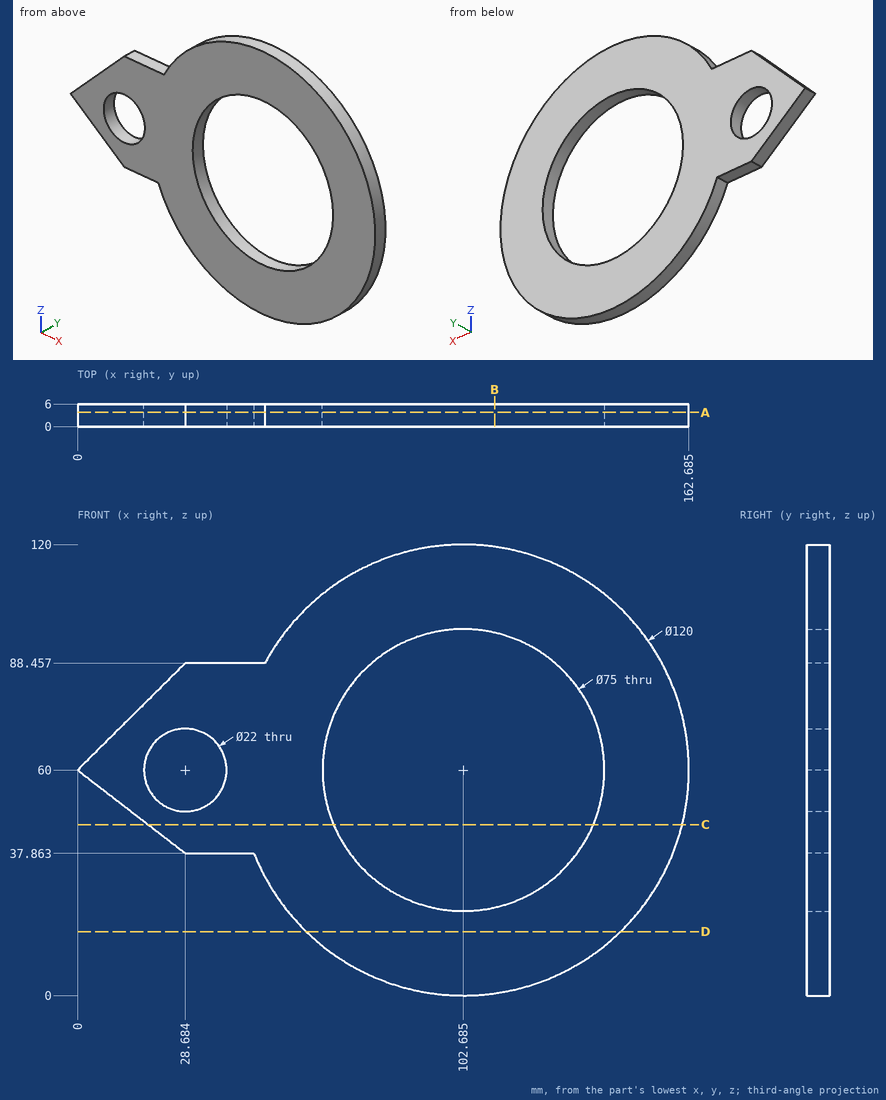
Geometry check sheet. Reference: drawing and pictorial views, mm from the part's lowest x, y, z. Coordinates: 2 decimals unless noted, no trailing zeros. Loops run counter-clockwise (first coordinate to the right, second up) from the corner with the lowest first, then second, coordinate; pieces in that order, holes last.
1) Sectioned sample at A-A (y = 3.8). Record the boundary of the cut face in (x, z) (1 decimal).
2) Sectioned sample at D-D (z = 17). Record the boundary of the cut face in (x, y), and give its area (3 significant figures).
3) Material ranges on probe 1 along X at (y, z) = (1.95, 60) (1 decimal); probe 2 along Z at (x, y) = (114, 2.95); probe 3 along Z at (x, y) = (98.5, 2.65) (1 decimal), recorded low to high.
4) Gauge pin test, flat ends, axial feed: pin 1 (1 mm diameter, centred on y = 5, z = 71.5, fed in from -X); pin 2 (1 mm diameter, centred on x = 118, z = 101, fed in from -Y); pin 3 (1.5 mm diameter, centred on y = 4, z = 101.5, fed in from -X) (1 decimal); pin 4 (1.5 mm diameter, centred on x = 73, y = 1, fed in from +Z). Record the tip position at first contact, or that the pin passes through.
5) Sectioned sample at B-B (x = 111). Record the boundary of the cut face in (y, z).
6) Sectioned sample at C-C (z = 45.5). Record the boundary of the cut face in (x, y), and give its area (3 significant figures).
Check sheet entries:
1. outline: (0, 60) - (28.7, 37.9) - (46.9, 37.9) arc R60 ccw (long way) to (49.9, 88.5) - (28.7, 88.5) - close; hole circle Ø22 at (28.7, 60); hole circle Ø75 at (102.7, 60)
2. outline: (60.84, 0) - (144.53, 0) - (144.53, 6) - (60.84, 6) - close
2. area: 502 mm2
3. probe 1: x = 0 to 17.7, 39.7 to 65.2, 140.2 to 162.7
3. probe 2: z = 1.08 to 24.25, 95.75 to 118.92
3. probe 3: z = 0.1 to 22.7, 97.3 to 119.9
4. pin 1: stops at x = 11.09
4. pin 2: stops at y = 0
4. pin 3: stops at x = 58.6
4. pin 4: stops at z = 112.56
5. outline: (0, 0.58) - (6, 0.58) - (6, 23.43) - (0, 23.43) - close; (0, 96.57) - (6, 96.57) - (6, 119.42) - (0, 119.42) - close
6. outline: (18.79, 0) - (68.1, 0) - (68.1, 6) - (18.79, 6) - close; (137.27, 0) - (160.91, 0) - (160.91, 6) - (137.27, 6) - close
6. area: 438 mm2
